The drawing under review shows one solid part. Ordinate dimensions are in mm from its lowest x, y, z. Round coordinates to 2 decimals unless told otherwise and drop trailing zeros. Order: outer loops, then holes, each group sorted by start corner. A loop starts at its lowest first (then second) coordinate and runs counter-clockwise, first axis right, second up. Notation, with made-up numbers: (-33, 0) -> (10, 0) arc R17 cw to (10, 9) -> close; hole circle Ø9 at (67, 85.25). An arc over 180 degrees is marked (long way). Use a Markdown table: item, result. Add a question column.
1) Consider section A-A (x = 14.75). State the section outline as (y, z) points, plus the area to 3 significant figures.
2) Consider section C-C (z = 7.25). State the section outline as (x, y) points, plus the area to 3 significant figures.
3) Wall thickness on line 1 along Y through (x, z) = (14.75, 5.5); line 2 along Y through (x, z) = (35.25, 4.75); line 3 along X through (y, z) = (4.5, 7.75): over which ranges is each line inside the solid? List them lowest first. Write a range as [from, to].
4) Consider section B-B (y = 20.25). State the section outline as (x, z) points.
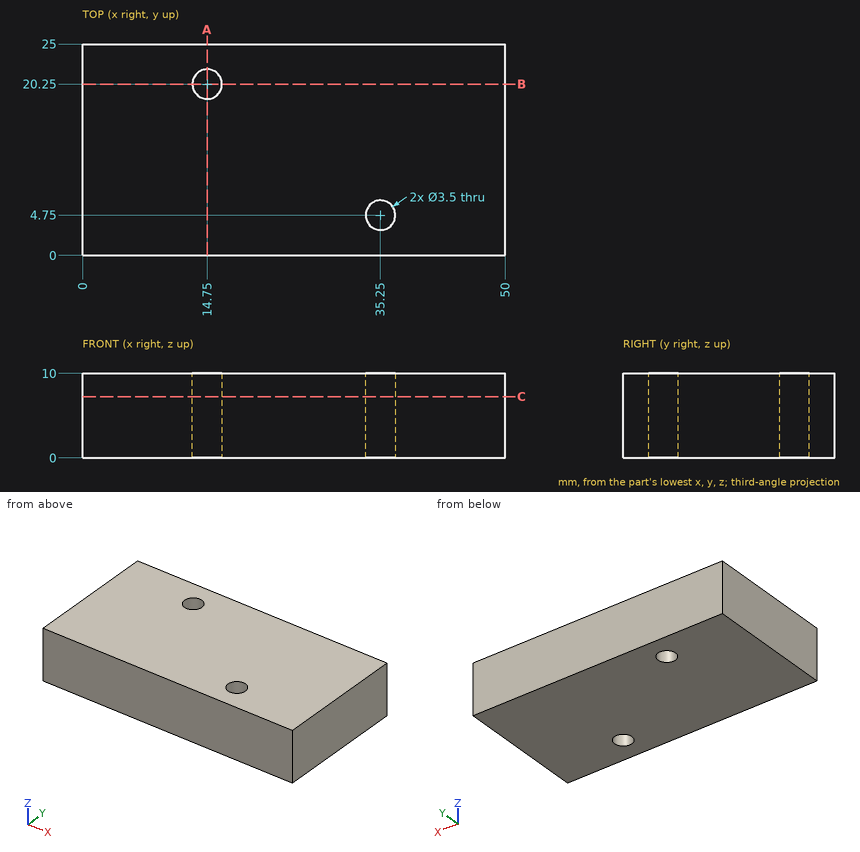
Results list:
| question | item | result |
|---|---|---|
| 1 | outline | (0, 0) -> (18.5, 0) -> (18.5, 10) -> (0, 10) -> close; (22, 0) -> (25, 0) -> (25, 10) -> (22, 10) -> close |
| 1 | area | 215 mm2 |
| 2 | outline | (0, 0) -> (50, 0) -> (50, 25) -> (0, 25) -> close; hole circle Ø3.5 at (14.75, 20.25); hole circle Ø3.5 at (35.25, 4.75) |
| 2 | area | 1,230 mm2 |
| 3 | line 1 | [0, 18.5], [22, 25] |
| 3 | line 2 | [0, 3], [6.5, 25] |
| 3 | line 3 | [0, 33.52], [36.98, 50] |
| 4 | outline | (0, 0) -> (13, 0) -> (13, 10) -> (0, 10) -> close; (16.5, 0) -> (50, 0) -> (50, 10) -> (16.5, 10) -> close |
